from build123d import *

# Parameters (mm, degrees)
CUT_EXTRUDE1_DEPTH  = 5
CIRPATTERN1_COUNT   = 5
SKETCH8_R           = 2.75
BOSS_EXTRUDE1_DEPTH = 6
CUT_EXTRUDE2_REACH  = 13


with BuildPart() as part:
    # Sketch3 → Shape_Roue (revolve)
    with BuildSketch(Plane.XY):
        Polygon((-2.5, 0), (2.5, 0), (2.5, 55), (6.5, 55), (6.5, 65), (-6.5, 65), (-6.5, 55), (-2.5, 55), align=None)
    revolve(axis=Axis((-2.5, 0, 0), (1, 0, 0)))

    # Sketch6 → Cut-Extrude1 (cut)
    with BuildSketch(Plane(origin=(2.5, 0, 0), x_dir=(0, 0, -1), z_dir=(1, 0, 0))):
        with BuildLine():
            Line((8.374067112, 8.374067112), (30.98386677, 30.98386677))
            ThreePointArc((30.98386677, 30.98386677), (33.994300587, 32.151296695), (36.886138794, 30.715025067))
            ThreePointArc((36.886138794, 30.715025067), (44.346217561, 18.368804754), (47.801241382, 4.363636364))
            ThreePointArc((47.801241382, 4.363636364), (46.772000384, 1.30320055), (43.8178046, 0))
            Line((43.8178046, 0), (11.842719282, 0))
            ThreePointArc((11.842719282, 0), (9.510338524, 0.750384638), (8.053049112, 2.72))
            ThreePointArc((8.053049112, 2.72), (7.852976026, 3.252809175), (7.617696081, 3.771035191))
            ThreePointArc((7.617696081, 3.771035191), (7.255426928, 6.194222796), (8.374067112, 8.374067112))
        make_face()
    cut_extrude1 = extrude(amount=-CUT_EXTRUDE1_DEPTH, mode=Mode.SUBTRACT)

    # CirPattern1: Cut-Extrude1 ×5 about axis
    cirpattern1_axis = Axis((0, 0, 0), (1, 0, 0))
    for i in range(1, CIRPATTERN1_COUNT):
        add(cut_extrude1.rotate(cirpattern1_axis, i * 360 / CIRPATTERN1_COUNT), mode=Mode.SUBTRACT)

    # Sketch8 → Boss-Extrude1 (add)
    with BuildSketch(Plane(origin=(-2.5, 0, 0), x_dir=(0, 0, -1), z_dir=(1, 0, 0))):
        Circle(SKETCH8_R)
    extrude(amount=-BOSS_EXTRUDE1_DEPTH)

    # Sketch7 → Cut-Extrude2 (cut, up to next)
    with BuildSketch(Plane(origin=(2.5, 0, 0), x_dir=(0, 0, -1), z_dir=(1, 0, 0)), mode=Mode.PRIVATE) as cut_extrude2_sk1:
        with BuildLine():
            Line((1.675, 1.307669683), (1.675, -1.307669683))
            ThreePointArc((1.675, -1.307669683), (-2.125, 0), (1.675, 1.307669683))
        make_face()
    cut_extrude2_tool1 = extrude(cut_extrude2_sk1.sketch, amount=-CUT_EXTRUDE2_REACH, mode=Mode.PRIVATE) & part.part
    add(cut_extrude2_tool1.solids().sort_by_distance((2.5, 0, 0.111388))[0], mode=Mode.SUBTRACT)


solid = part.part
Source: CAD feature listing. Evaluate the final solid. Frame: model axes, mm. A direction names the side the tool comes from. Coordinates: 2 decimals unless noted, no trailing zeros. Loops run counter-clockwise (first coordinate to the right, second up) from the corner with the lowest first, then second, coordinate; pieces in that order, holes last. Notation, with made-up numbers: (48, 55) - (72, 55) arc R22 cw to (72, 93) - close; hole circle Ø7 at (-14, 37). An arc over 180 degrees is marked (long way). One line per question, with ' | ' between items.
1) First-contact query: P1, Ø1, axis at x = -6, z = -43, coming from the +Y side; P2, Ø6, axis at y = -41.5, z = 2.5, coming from the +X side; P3, Ø2, axis at x = 1.5, z = -20, coming from the +Y side. Flat tips, straight axial feed; report the tip coordinate or a pass-through.
Report:
P1: stops at y = 49.18 | P2: stops at x = 2.5 | P3: stops at y = 62.16
2) Section C-C, the plane y = -57. Return loops of the section in (x, z), then the cut area to 3 significant figures.
Report:
outline: (-6.5, -31.24) - (6.5, -31.24) - (6.5, 31.24) - (-6.5, 31.24) - close | area: 812 mm²
3) Section A-A, the plane z = 27.5. Return loops of the section in (x, y), then the cut area to 3 significant figures.
Report:
outline: (-6.5, -58.9) - (6.5, -58.9) - (6.5, -47.63) - (2.5, -47.63) - (2.5, -39.34) - (-2.5, -39.34) - (-2.5, -47.63) - (-6.5, -47.63) - close; (-6.5, 47.63) - (-2.5, 47.63) - (-2.5, 19.98) - (2.5, 19.98) - (2.5, 47.63) - (6.5, 47.63) - (6.5, 58.9) - (-6.5, 58.9) - close; (-2.5, -19.98) - (2.5, -19.98) - (2.5, -4.36) - (-2.5, -4.36) - close | area: 551 mm²
4) Set-up query: faces 1 (the face through (0.04, -22.35, -41.07)), 2 (the face through (-4.472, -11.923, -53.692)), 3 (the face through (4.528, -11.923, -53.692)). Return all of +Z, -Z, +X, -X, +Y, -Y with unobstructed straight access to the full face (end or side cutting, diameter ignored); none if empty.
Report:
face 1: +X, -X | face 2: -X | face 3: +X
5) Pull-direction query (Y, two-part tool) for faces 4 (the face through (-0.09, 62, 19.52)), 5 (the face through (0.035, 9.298, -2.253)); classes: released by +Y, released by -Y, zero draft, split by the parting line, or undercut.
Report:
face 4: split by the parting line | face 5: undercut
6) Section B-B, the plane x = 4.75. Return loops of the section in (y, z).
Report:
outline: circle Ø130 at (0, 0); hole circle Ø110 at (0, 0)
7) Line query: line 1 along Y through (x, z) = (0.75, 35); line 2 along Z through (x, y) = (-2.25, 1) (3 decimals); line 3 along Z through (x, y) = (-1.75, -29). Output: solid intervals per line, ascending.
Report:
line 1: y = -54.77 to -32.85, -25.43 to -5.54, 25.43 to 54.77 | line 2: z = -64.992 to -46.464, -9.197 to -1.675, 1.875 to 8.476, 47.99 to 64.992 | line 3: z = -58.17 to -38.25, -9.42 to 4.59, 37.1 to 58.17
